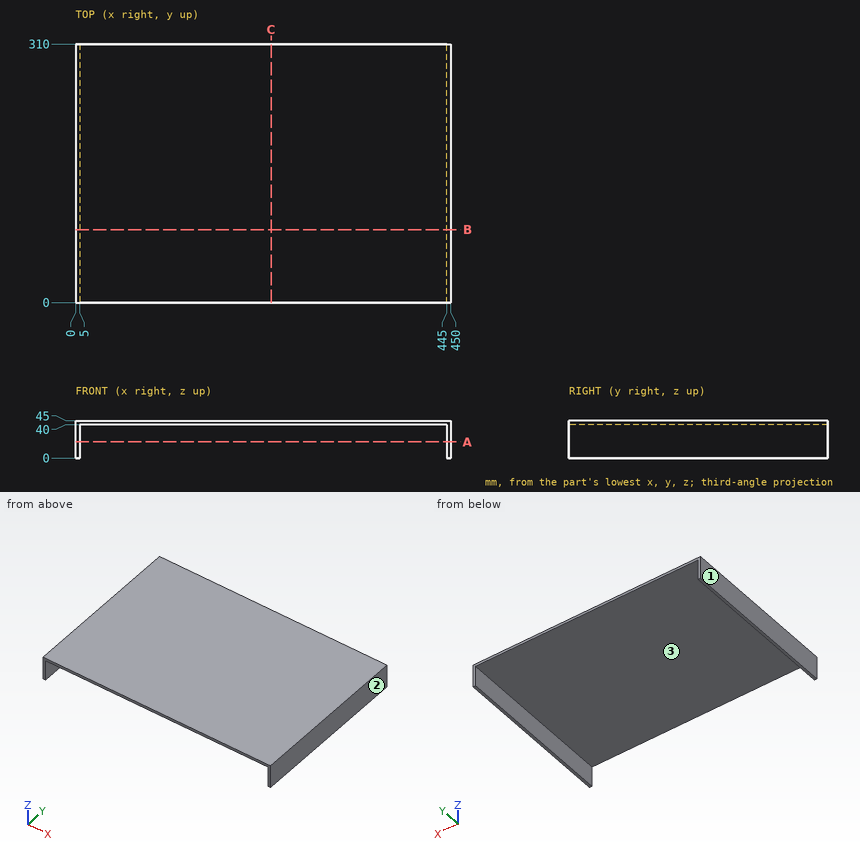
Source: three-view drawing plus pictorial views. Frame: mm from the lowest corner of the part. Round coordinates to 2 decimals unless told otherwise and drop trailing zeros. Loops run counter-clockwise (first coordinate to the right, second up) from the corner with the lowest first, then second, coordinate; pieces in that order, holes last. Notation, with made-up numbers: M 53,88.25 L 102,88.25 A30 cw 102,112.25 Z; hole C 3.25,77 d1. An arc over 180 degrees is marked long. Put each result on its own line as item: value.
(1) Section B-B, the plane y = 87.5. Return loops of the section in (x, z).
Solutions:
outline: M 0,0 L 5,0 L 5,40 L 445,40 L 445,0 L 450,0 L 450,45 L 0,45 Z
(2) First-contact query: pin 1 (8 mm diameter, centred on x = 92.5, y = 273, fed in from -Z). Flat tip, straight axial feed; report the tip coordinate or a pass-through.
Solutions:
pin 1: z = 40
(3) Ray query, line 1 (X direction, y = 28, z = 16.5); line 2 (Z direction, x = 114, y = 204). Return the intervals inside material, ascending. Write a range as [from, to].
Solutions:
line 1: [0, 5], [445, 450]
line 2: [40, 45]
(4) Section A-A, the plane z = 19.5. Return loops of the section in (x, y), and give its area (3 significant figures).
Solutions:
outline: M 0,0 L 5,0 L 5,310 L 0,310 Z; M 445,0 L 450,0 L 450,310 L 445,310 Z
area: 3,100 mm²
(5) Pull-direction query (X, two-part tool) for the marked faces 1, 2 and 3; classes: released by +X, released by -X, zero draft, split by the parting line, or undercut.
Solutions:
face 1: released by -X
face 2: released by +X
face 3: undercut
(6) Section C-C, the plane x = 234.5. Return loops of the section in (y, z).
Solutions:
outline: M 0,40 L 310,40 L 310,45 L 0,45 Z
